Here's how the part is built. I have some questions about the finished solid (model axes, mm). A direction names the side the tool comes from. Coordinates: 2 decimals unless noted, no trailing zeros. Order: outer loops, then holes, each group sorted by start corner. A loop starts at its lowest first (then second) coordinate and runs counter-clockwise, first axis right, second up.
```python
from build123d import *

# Parameters (mm, degrees)
SKETCH_1_R      = 1.525
SKETCH_1_R_2    = 2.75
EXTRUDE_1_DEPTH = 13
EXTRUDE_2_DEPTH = 4
FILLET_1_R      = 8
FILLET_2_R      = 1
FILLET_3_R      = 10


with BuildPart() as part:
    # 草图1 → 凸台-拉伸1 (new body)
    with BuildSketch(Plane(origin=(0, 0, 0), x_dir=(1, 0, 0), z_dir=(0, 1, 0))):
        with BuildLine():
            Line((-10, 0), (0, 0))
            Line((0, 0), (5, 0))
            Line((5, 0), (5, 15))
            Line((5, 15), (15, 15))
            Line((15, 15), (15, 0))
            Line((15, 0), (20, 0))
            Line((20, 0), (20, 20))
            Line((20, 20), (0, 20))
            Line((0, 20), (-10, 20))
            ThreePointArc((-10, 20), (-20, 10), (-10, 0))
        make_face()
        with Locations(Location((-10, 3.25, 0), (0, 0, 90))):
            Circle(SKETCH_1_R, mode=Mode.SUBTRACT)
        with Locations(Location((-16.75, 10, 0), (0, 0, 90))):
            Circle(SKETCH_1_R, mode=Mode.SUBTRACT)
        with Locations(Location((-10, 10, 0), (0, 0, 90))):
            Circle(SKETCH_1_R_2, mode=Mode.SUBTRACT)
        with Locations(Location((-10, 16.75, 0), (0, 0, 90))):
            Circle(SKETCH_1_R, mode=Mode.SUBTRACT)
        with Locations(Location((-3.25, 10, 0), (0, 0, 90))):
            Circle(SKETCH_1_R, mode=Mode.SUBTRACT)
    extrude(amount=EXTRUDE_1_DEPTH)

    # 草图1<3> → 凸台-拉伸2 (add)
    with BuildSketch(Plane(origin=(0, 0, 0), x_dir=(1, 0, 0), z_dir=(0, 1, 0))):
        Polygon((5, 0), (0, 0), (0, -20), (20, -20), (20, 0), (15, 0), (15, 15), (5, 15), align=None)
        with BuildLine():
            Line((8.7, -17), (8.7, 4.846192362))
            ThreePointArc((8.7, 4.846192362), (10, 6.146192362), (11.3, 4.846192362))
            Line((11.3, 4.846192362), (11.3, -17))
            ThreePointArc((11.3, -17), (10, -18.3), (8.7, -17))
        make_face(mode=Mode.SUBTRACT)
    extrude(amount=EXTRUDE_2_DEPTH)

    # 圆角1
    fillet_1_edges = [part.edges().sort_by_distance(p)[0] for p in [
        (0, 2, 0),
    ]]
    fillet(fillet_1_edges, radius=FILLET_1_R)

    # 圆角2
    fillet_2_edges = [part.edges().sort_by_distance(p)[0] for p in [
        (17.5, 4, 0),
        (15, 4, -7.5),
        (10, 4, -15),
        (5, 4, -7.5),
        (-1.5, 4, 0),
    ]]
    fillet(fillet_2_edges, radius=FILLET_2_R)

    # 圆角3
    fillet_3_edges = [part.edges().sort_by_distance(p)[0] for p in [
        (20, 2, 20),
        (0, 2, 20),
    ]]
    fillet(fillet_3_edges, radius=FILLET_3_R - 0.0001)  # a hair under: the kernel refuses the full size


solid = part.part
```
Q1. If we section it at B-B on z = -10: Write out the boundary of the cut face in (x, y) (3 decimals), then the cut area to 3 significant figures.
Q2. If we section it at C-C on x = -16.75: Write out the boundary of the cut face in (y, z) (3 decimals), then the cut area to 3 significant figures.
Q3. I need wall thicknesses on L1, parallel to X at y = 3.75, z = -10 (3 decimals); L2, parallel to Z at x = -10, y = 9.75 (3 decimals); L3, parallel to X at y = 6.25, z = -10 (3 decimals). Which ranges of each line are inside material? Lowest first, please.
Q4. Will these pins go through, and if not, where does the flat tip stop? pin 1 (7 mm diameter, centred on x = 6.5, z = 6.5, fed in from +Y); pin 2 (2.5 mm diameter, centred on y = 8, z = -10.5, fed in from -X); pin 3 (1.6 mm diameter, centred on y = 2, z = 8.5, fed in from -X); pin 4 (1.5 mm diameter, centred on x = 17, y = 8.5, fed in from +Z).
Q5. For faces 1 (the flat face through (5, 6, -20)), 2 (the cylindrical face through (14.699, 4.285, -7.112)), 3 (the cylindrical face through (9.971, 1.972, -6.146)), 4 (the flat face through (4, 0, -5)), 5 (the flat face through (0, 2, 9)), which set-ups out of +Z, -Z, +X, -X, +Y, -Y let a thin tool reach every point of the face, with its end or its side?
Q6. If we section it at D-D on z = -5.5: Write out the boundary of the cut face in (x, y).
Q7. We'd pull the mould along X, two halves only. Please class faces 6 (the cylindrical face through (-20, 6, -10)), 7 (the cylindrical face through (16.99, 2.03, 17.15)), 8 (the flat face through (5, 9, -7)), 9 (the flat face through (17, 9, 0)): pulls with the +X half, pulls with the -X half, needs draft (parallel to the pull), parting line crosses it, or undercut.
Q8. If we section it at A-A on y = 6.25: Write out the boundary of the cut face in (x, z) (3 decimals), then the cut area to 3 significant figures.
Reply:
1. outline: (-20, 0) - (-18.275, 0) - (-18.275, 13) - (-20, 13) - close; (-15.225, 0) - (-12.75, 0) - (-12.75, 13) - (-15.225, 13) - close; (-7.25, 0) - (-4.775, 0) - (-4.775, 13) - (-7.25, 13) - close; (-1.725, 0) - (20, 0) - (20, 13) - (15, 13) - (15, 5) arc R1 cw to (14, 4) - (6, 4) arc R1 cw to (5, 5) - (5, 13) - (-1.725, 13) - close
1. area: 280 mm2
2. outline: (0, -17.378) - (13, -17.378) - (13, -11.525) - (0, -11.525) - close; (0, -8.475) - (13, -8.475) - (13, -2.622) - (0, -2.622) - close
2. area: 152 mm2
3. L1: x = -20 to -18.275, -15.225 to -12.75, -7.25 to -4.775, -1.725 to 20
3. L2: z = -20 to -18.275, -15.225 to -12.75, -7.25 to -4.775, -1.725 to 0
3. L3: x = -20 to -18.275, -15.225 to -12.75, -7.25 to -4.775, -1.725 to 5, 15 to 20
4. pin 1: stops at y = 4
4. pin 2: stops at x = -20
4. pin 3: stops at x = -0.01
4. pin 4: stops at z = 0
5. face 1: -Z, +X, -X, +Y, -Y
5. face 2: +Z, +Y
5. face 3: +Y, -Y
5. face 4: +Z, -Z, +X, -X, -Y
5. face 5: +Z, -X, +Y, -Y
6. outline: (-18.93, 0) - (8.88, 0) - (8.88, 4) - (6, 4) arc R1 cw to (5, 5) - (5, 13) - (-18.93, 13) - close; (11.12, 0) - (20, 0) - (20, 13) - (15, 13) - (15, 5) arc R1 cw to (14, 4) - (11.12, 4) - close
7. face 6: pulls with the -X half
7. face 7: pulls with the +X half
7. face 8: undercut
7. face 9: needs draft
8. outline: (-10, -20) - (20, -20) - (20, 0) - (15, 0) - (15, -15) - (5, -15) - (5, 0) - (-10, 0) arc R10 ccw to start; hole circle Ø3.05 at (-16.75, -10); hole circle Ø5.5 at (-10, -10); hole circle Ø3.05 at (-10, -16.75); hole circle Ø3.05 at (-10, -3.25); hole circle Ø3.05 at (-3.25, -10)
8. area: 554 mm2
